Check sheet for the modelled part. Datum: model origin and axes. Units: mm. Face numbers are marked on the shaded views. A direction names the side the tool comes from. Give positions to 0.01 mm unless a question says otherwise; leave off trailing zeros. Write each loop counter-clockwise with the first axis right and the second up, starting at its lowest first coordinate (ties: lowest second). Pieces come first, ordered by that corner, then holes. Notation, with made-up numbers: M 38.25,77 L 68.25,77 A30 cw 68.25,115 Z; hole C 40,32.25 d1. An arc over 180 degrees is marked long. Write item = value, one per line. Start each with the question number.
1) Sectioned sample at D-D, the plane x = -4.5. Record the cut outline in (y, z), then the cut area to 3 significant figures.
2) Gauge pin test, flat ends, axial feed: pin 1 (2.5 mm diameter, centred on x = 0.5, z = 7, fed in from +Y); pin 2 (1 mm diameter, centred on x = 4, z = 1, fed in from +Y); pin 3 (1 mm diameter, centred on x = 0, y = 15, fed in from +Z). Record the tip position at first contact, or that the pin passes through.
3) Sectioned sample at C-C, the plane y = 16.25. Record the cut outline in (x, z), then the cut area to 3 significant figures.
4) Scan lines: L1, parallel to Y at x = 5.75, z = 0.5; L2, parallel to Y at x = 0, z = 0; L3, parallel to Z at x = 1, y = 18.75. Record each from-to range of solid material in increasing order.
5) Draft check along X on the marked faces 1, 2, 3 and 4. Enter one of: pulls with the +X half, pulls with the -X half, needs draft (parallel to the pull), parting line crosses it, or undercut.
6) Sectioned sample at B-B, the plane z = 0. Record the cut outline in (x, y).
7) Set-up check for the marked faces 5, 6, 7 and 8: record each of +Z, -Z, +X, -X, +Y, -Y from which the full face is reachable in a straight line by a thin tool's end or side.
8) Sectioned sample at A-A, the plane x = 5.01. Record the cut outline in (y, z).
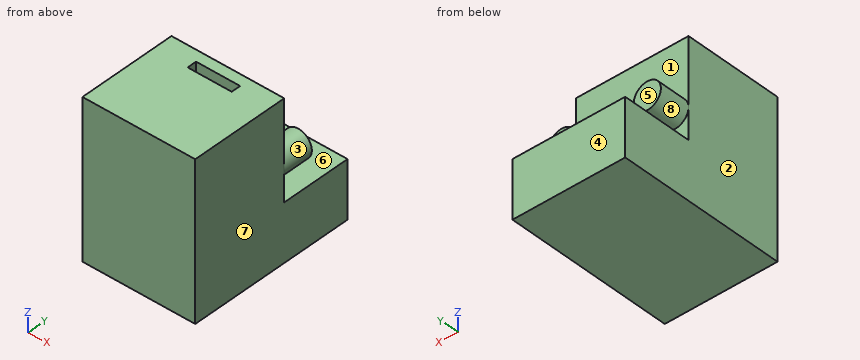
from build123d import *

# Parameters (mm, degrees)
SKETCH1_W           = 13.2
SKETCH1_H           = 18.2
BOSS_EXTRUDE1_DEPTH = 11.6
SKETCH2_R           = 1.59
BOSS_EXTRUDE2_DEPTH = 3.6
SKETCH3_W           = 13.2
SKETCH3_H           = 6.7
BOSS_EXTRUDE3_DEPTH = 8.25
SKETCH4_W           = 5.164958048
SKETCH4_H           = 1.096471541
CUT_EXTRUDE1_DEPTH  = 5


with BuildPart() as part:
    # Sketch1 → Boss-Extrude1 (new body)
    with BuildSketch(Plane(origin=(0, 0, 0), x_dir=(1, 0, 0), z_dir=(0, 1, 0))):
        Rectangle(SKETCH1_W, SKETCH1_H)
    extrude(amount=BOSS_EXTRUDE1_DEPTH)

    # Sketch2 → Boss-Extrude2 (add)
    with BuildSketch(Plane(origin=(0, 11.6, 0), x_dir=(1, 0, 0), z_dir=(0, 1, 0))):
        with Locations((-5.01, -1.24)):
            Circle(SKETCH2_R)
    boss_extrude2 = extrude(amount=BOSS_EXTRUDE2_DEPTH)

    # Mirror1: Boss-Extrude2 across plane
    add(boss_extrude2.mirror(Plane(origin=(0, 0, 0), x_dir=(0, 0, 1), z_dir=(1, 0, 0))))

    # Sketch3 → Boss-Extrude3 (add)
    with BuildSketch(Plane(origin=(0, 11.6, 0), x_dir=(1, 0, 0), z_dir=(0, 1, 0))):
        with Locations((0, 5.75)):
            Rectangle(SKETCH3_W, SKETCH3_H)
    extrude(amount=BOSS_EXTRUDE3_DEPTH)

    # Sketch4 → Cut-Extrude1 (cut)
    with BuildSketch(Plane.XY.offset(9.1)):
        with Locations((0, 9.780727429)):
            Rectangle(SKETCH4_W, SKETCH4_H)
    extrude(amount=-CUT_EXTRUDE1_DEPTH, mode=Mode.SUBTRACT)


solid = part.part
Data:
q1.outline = M 0,-9.1 L 19.85,-9.1 L 19.85,-2.4 L 11.6,-2.4 L 11.6,-0.27 L 15.2,-0.27 L 15.2,2.75 L 11.6,2.75 L 11.6,9.1 L 0,9.1 Z
q1.area = 277 mm2
q2.pin_1 = 11.6
q2.pin_2 = 15.2
q2.pin_3 = -2.4
q3.outline = M -6.6,-9.1 L 6.6,-9.1 L 6.6,-2.4 L -6.6,-2.4 Z
q3.area = 88.4 mm2
q4.L1 = 0 to 15.2
q4.L2 = 0 to 11.6
q4.L3 = -9.1 to -2.4
q5.face_1 = undercut
q5.face_2 = pulls with the -X half
q5.face_3 = undercut
q5.face_4 = needs draft
q6.outline = M -6.6,0 L 6.6,0 L 6.6,11.6 L 6.01,11.6 L 6.01,15.2 L 4.01,15.2 L 4.01,11.6 L -4.01,11.6 L -4.01,15.2 L -6.01,15.2 L -6.01,11.6 L -6.6,11.6 Z
q7.face_5 = +Z, +X, -X, +Y
q7.face_6 = +X, -X, +Y
q7.face_7 = +Z, -Z, +X, +Y, -Y
q7.face_8 = +Y
q8.outline = M 0,-9.1 L 19.85,-9.1 L 19.85,-2.4 L 11.6,-2.4 L 11.6,-0.35 L 15.2,-0.35 L 15.2,2.83 L 11.6,2.83 L 11.6,9.1 L 0,9.1 Z
